Design review of the part built by this model. Coordinates are the model's own, in mm. Face numbers are marked on the shaded views. A direction names the side the tool comes from. Coordinates: 2 decimals unless noted, no trailing zeros. Loops run counter-clockwise (first coordinate to the right, second up) from the corner with the lowest first, then second, coordinate; pieces in that order, holes last. Notation, with made-up numbers: (4.5, 37.25) -> (47.5, 37.25) arc R20 ccw to (47.5, 59.25) -> close; hole circle Ø9 at (18.5, -37). An arc over 180 degrees is marked (long way). Answer in a Markdown table with one row per item.
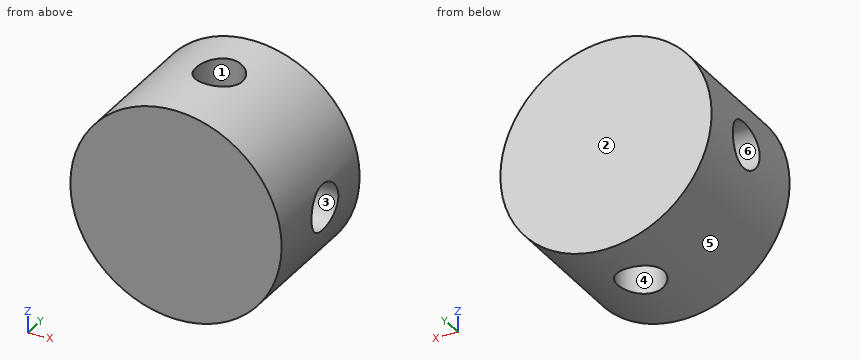
```python
from build123d import *

# Parameters (mm, degrees)
SKETCH1_R           = 14.1
BOSS_EXTRUDE1_DEPTH = 18
SKETCH2_R           = 3.1
CUT_EXTRUDE1_DEPTH  = 9
CIRPATTERN1_COUNT   = 4


with BuildPart() as part:
    # Sketch1 → Boss-Extrude1 (new body)
    with BuildSketch(Plane(origin=(0, 0, 0), x_dir=(1, 0, 0), z_dir=(0, 1, 0))):
        with Locations(Location((0, 0, 0), (0, 0, 270))):
            Circle(SKETCH1_R)
    extrude(amount=BOSS_EXTRUDE1_DEPTH)

    # Sketch2 → Cut-Extrude1 (cut)
    with BuildSketch(Plane(origin=(14.1, 0, 0), x_dir=(0, 0, -1), z_dir=(1, 0, 0))):
        with Locations((0, 9.995362646)):
            Circle(SKETCH2_R)
    cut_extrude1 = extrude(amount=-CUT_EXTRUDE1_DEPTH, mode=Mode.SUBTRACT)

    # CirPattern1: Cut-Extrude1 ×4 about axis
    cirpattern1_axis = Axis((0, 0, 0), (0, 1, 0))
    for i in range(1, CIRPATTERN1_COUNT):
        add(cut_extrude1.rotate(cirpattern1_axis, i * 360 / CIRPATTERN1_COUNT), mode=Mode.SUBTRACT)


solid = part.part
```
(1) Draft analysis for pull direction Z (two halves, no side actions). For the marked faces 4, 5 and 6, state which applies: pulls with the +Z half, pulls with the -Z half, needs draft (parallel to the pull), parting line crosses it, or undercut.
Evaluation:
| item | result |
|---|---|
| face 4 | needs draft |
| face 5 | parting line crosses it |
| face 6 | undercut |
(2) Take a section at C-C on z = 8.5. Give the boundary of the cut face in (x, y).
Evaluation:
| item | result |
|---|---|
| outline | (-11.25, 0) -> (11.25, 0) -> (11.25, 18) -> (-11.25, 18) -> close; hole circle Ø6.2 at (0, 10) |
(3) To check wall thickness, follow probe 1 along Y at (x, z) = (11.5, 0); probe 2 along X at (y, z) = (8, -2); probe 3 along X at (y, z) = (11.75, 7.75). State the ranges of each line that lie inside material, in increasing order.
Evaluation:
| item | result |
|---|---|
| probe 1 | y = 0 to 6.9, 13.1 to 18 |
| probe 2 | x = -5.1 to 5.1 |
| probe 3 | x = -11.78 to -2.56, 2.56 to 11.78 |
(4) Take a section at D-D on x = 0. Give the boundary of the cut face in (y, z).
Evaluation:
| item | result |
|---|---|
| outline | (0, -14.1) -> (6.9, -14.1) -> (6.9, -5.1) -> (13.1, -5.1) -> (13.1, -14.1) -> (18, -14.1) -> (18, 14.1) -> (13.1, 14.1) -> (13.1, 5.1) -> (6.9, 5.1) -> (6.9, 14.1) -> (0, 14.1) -> close |
(5) Tool access review of the marked faces 1, 2 and 3: name each direction out of +Z, -Z, +X, -X, +Y, -Y from which nothing blocks a thin tool from reaching the whole face with its end or side.
Evaluation:
| item | result |
|---|---|
| face 1 | +Z |
| face 2 | +Z, -Z, +X, -X, +Y |
| face 3 | +X |
(6) Take a section at B-B on x = -12. Give the boundary of the cut face in (y, z).
Evaluation:
| item | result |
|---|---|
| outline | (0, -7.4) -> (18, -7.4) -> (18, 7.4) -> (0, 7.4) -> close; hole circle Ø6.2 at (10, 0) |
(7) Take a section at A-A on z = 0. Give the boundary of the cut face in (x, y).
Evaluation:
| item | result |
|---|---|
| outline | (-14.1, 0) -> (14.1, 0) -> (14.1, 6.9) -> (5.1, 6.9) -> (5.1, 13.1) -> (14.1, 13.1) -> (14.1, 18) -> (-14.1, 18) -> (-14.1, 13.1) -> (-5.1, 13.1) -> (-5.1, 6.9) -> (-14.1, 6.9) -> close |
(8) For pin 1 (5.5 mm diameter, centred on y = 10, z = 0, fed in from +X); pin 2 (10 mm diameter, centred on x = 0, y = 10, fed in from -Z); pin 3 (3 mm diameter, centred on y = 9.5, z = 0, fed in from -X); pin 4 (10 mm diameter, centred on y = 10.5, z = -10, fed in from +X), all flat-tipped, find the tip position at first contact; note any pin that passes through.
Evaluation:
| item | result |
|---|---|
| pin 1 | stops at x = 5.1 |
| pin 2 | stops at z = -14.1 |
| pin 3 | stops at x = -5.1 |
| pin 4 | stops at x = 13.18 |
